Design review of the part built by this model. Coordinates are the model's own, in mm. A direction names the side the tool comes from. Coordinates: 2 decimals unless noted, no trailing zeros. Write each loop counter-clockwise with the first axis right and the second up, starting at its lowest first coordinate (ties: lowest second). Pieces come first, ordered by that corner, then holes. Notation, with made-up numbers: (63.25, 18) -> (84.25, 18) arc R21 ccw to (84.25, 43) -> close; hole circle Ø1 at (81, 89). An arc over 180 degrees is marked (long way). Return JSON: item names as keys, results as strings. Group by question number.
from build123d import *

# Parameters (mm, degrees)
CYLINDER095_R      = 1.5
CYLINDER095_DEPTH  = 21
CYLINDER094_R      = 1.5
CYLINDER094_DEPTH  = 21
CYLINDER085_R      = 1.5
CYLINDER085_DEPTH  = 12
CYLINDER088_R      = 3
CYLINDER088_DEPTH  = 1
CYLINDER089_R      = 3
CYLINDER089_DEPTH  = 1
CYLINDER087_R      = 5.5
CYLINDER087_DEPTH  = 4
CYLINDER086_R      = 5.5
CYLINDER086_DEPTH  = 4
BOX406008013_W     = 15
BOX406008013_H     = 29
BOX406008013_DEPTH = 18
CHAMFER_SIZE       = 0.5
CHAMFER001_SIZE    = 0.5


with BuildPart() as cylinder095:
    # Cylinder095 → Cylinder095 (new body)
    with BuildSketch(Plane(origin=(3, -13, -4), x_dir=(1, 0, 0), z_dir=(0, -1, 0))):
        Circle(CYLINDER095_R)
    extrude(amount=CYLINDER095_DEPTH)


with BuildPart() as fusion103077013004017014:
    # Cylinder094 → Cylinder094 (new body)
    with BuildSketch(Plane(origin=(-3, -13, -14), x_dir=(1, 0, 0), z_dir=(0, -1, 0))):
        Circle(CYLINDER094_R)
    extrude(amount=CYLINDER094_DEPTH)

    # Fusion103077013004017014: union Cylinder095
    add(cylinder095.part)


with BuildPart() as cylinder081:
    # Cylinder085 → Cylinder085 (new body)
    with BuildSketch(Plane.XY.offset(-14)):
        Circle(CYLINDER085_R)
    extrude(amount=CYLINDER085_DEPTH)


with BuildPart() as cylinder082:
    # Cylinder088 → Cylinder088 (new body)
    with BuildSketch(Plane.XY.offset(-5)):
        Circle(CYLINDER088_R)
    extrude(amount=CYLINDER088_DEPTH)


with BuildPart() as fusion103077013004017009:
    # Cylinder089 → Cylinder089 (new body)
    with BuildSketch(Plane.XY.offset(-14)):
        Circle(CYLINDER089_R)
    extrude(amount=CYLINDER089_DEPTH)

    # Fusion103077013004017009: union Cylinder082
    add(cylinder082.part)


with BuildPart() as f_623_bearing003:
    # Cylinder087 → Cylinder087 (new body)
    with BuildSketch(Plane.XY.offset(-18)):
        Circle(CYLINDER087_R)
    extrude(amount=CYLINDER087_DEPTH)


with BuildPart() as f_623_bearing_holes:
    # Cylinder086 → Cylinder086 (new body)
    with BuildSketch(Plane.XY.offset(-4)):
        Circle(CYLINDER086_R)
    extrude(amount=CYLINDER086_DEPTH)

    # Fusion103077013004017008: union 623 Bearing003
    add(f_623_bearing003.part)


with BuildPart() as bearing_mount_end:
    # Box406008013 → Box406008013 (new body)
    with BuildSketch(Plane(origin=(-7.5, -22, -18), x_dir=(1, 0, 0), z_dir=(0, 0, 1))):
        with Locations((7.5, 14.5)):
            Rectangle(BOX406008013_W, BOX406008013_H)
    extrude(amount=BOX406008013_DEPTH)

    # Cut070: cut 623 Bearing Holes
    add(f_623_bearing_holes.part, mode=Mode.SUBTRACT)

    # Cut071: cut Fusion103077013004017009
    add(fusion103077013004017009.part, mode=Mode.SUBTRACT)

    # Cut072: cut Cylinder081
    add(cylinder081.part, mode=Mode.SUBTRACT)

    # Chamfer
    chamfer_edges = [bearing_mount_end.edges().sort_by_distance(p)[0] for p in [
        (-3, 0, -5),
    ]]
    chamfer(chamfer_edges, length=CHAMFER_SIZE)

    # Chamfer001
    chamfer001_edges = [bearing_mount_end.edges().sort_by_distance(p)[0] for p in [
        (-3, 0, -13),
    ]]
    chamfer(chamfer001_edges, length=CHAMFER001_SIZE)

    # Cut078: cut Fusion103077013004017014
    add(fusion103077013004017014.part, mode=Mode.SUBTRACT)


solid = bearing_mount_end.part
Q1. We need section A-A on y = 0. Write out the cut boundary in (x, z), plus the area to 4 significant figures.
Q2. We need section C-C on z = -3. Write out the cut boundary in (x, y), plus the area to 3 significant figures.
Q3. We need section D-D on z = -7.25. Write out the cut boundary in (x, y), plus the area to 3 significant figures.
Q4. For faces 1 (the flat face through (0, -11, 0)), 2 (the flat face through (2.4, -2.4, -14)), 3 (the flat face through (-3, -13, -14)), 4 (the flat face through (2.4, -2.4, -4)), list the 3-axis set-ups (+Z, -Z, +X, -X, +Y, -Y) from which the entire face can be reached by the end or side of a thin tool; tool diameter is ignored.
Q5. Wall thickness on L1, parallel to Z at x = -3, y = -20.25; L2, parallel to X at y = -18.25, z = -14; L3, parallel to X at y = -15.25, z = -4: over which ranges is each line inside the solid? List them lowest first.
Q6. The part is to be moulded in two halves that separate along X. For faces 5 (the flat face through (-7.5, -8, -9)), 6 (the flat face through (0, -22, -9)), 7 (the cylindrical face through (-1.5, 0.07, -9.06)), 8 (the flat face through (7.5, -8, -9)), say which applies: +X half, -X half, draft (parallel to the pull), parting line (faces both ways), or undercut.
Q7. For P1, Ø5.5, axis at x = 0, y = -1, coming from the -Z side; P2, Ø5.5, axis at x = 1, y = 0, coming from the +Z side; P3, Ø0.9, axis at x = 3.5, z = -4.5, coming from the -Y side, all flat-tipped, find the tip position at first contact; note any pin that passes through.
Q8. We need section B-B on x = 0. Write out the cut boundary in (y, z).
Findings below:
{
 "1": {"outline": "(-7.5, -18) -> (-5.5, -18) -> (-5.5, -14) -> (-3, -14) -> (-3, -13.5) -> (-2.5, -13) -> (-1.5, -13) -> (-1.5, -5) -> (-2.5, -5) -> (-3, -4.5) -> (-3, -4) -> (-5.5, -4) -> (-5.5, 0) -> (-7.5, 0) -> close; (1.5, -13) -> (2.5, -13) -> (3, -13.5) -> (3, -14) -> (5.5, -14) -> (5.5, -18) -> (7.5, -18) -> (7.5, 0) -> (5.5, 0) -> (5.5, -4) -> (3, -4) -> (3, -4.5) -> (2.5, -5) -> (1.5, -5) -> close", "area": "146.5 mm^2"},
 "2": {"outline": "(-7.5, -22) -> (1.88, -22) -> (1.88, -13) -> (4.12, -13) -> (4.12, -22) -> (7.5, -22) -> (7.5, 7) -> (-7.5, 7) -> close; hole circle Ø11 at (0, 0)", "area": "320 mm^2"},
 "3": {"outline": "(-7.5, -22) -> (7.5, -22) -> (7.5, 7) -> (-7.5, 7) -> close; hole circle Ø3 at (0, 0)", "area": "428 mm^2"},
 "4": {"face 1": "+Z, +X, -X, +Y, -Y", "face 2": "-Z", "face 3": "-Y", "face 4": "+Z"},
 "5": {"L1": "z = -18 to -15.5, -12.5 to 0", "L2": "x = -7.5 to -4.5, -1.5 to 7.5", "L3": "x = -7.5 to 1.5, 4.5 to 7.5"},
 "6": {"face 5": "-X half", "face 6": "draft", "face 7": "undercut", "face 8": "+X half"},
 "7": {"P1": "stops at z = -14", "P2": "stops at z = -4", "P3": "stops at y = -13"},
 "8": {"outline": "(-22, -18) -> (-5.5, -18) -> (-5.5, -14) -> (-3, -14) -> (-3, -13.5) -> (-2.5, -13) -> (-1.5, -13) -> (-1.5, -5) -> (-2.5, -5) -> (-3, -4.5) -> (-3, -4) -> (-5.5, -4) -> (-5.5, 0) -> (-22, 0) -> close; (1.5, -13) -> (2.5, -13) -> (3, -13.5) -> (3, -14) -> (5.5, -14) -> (5.5, -18) -> (7, -18) -> (7, 0) -> (5.5, 0) -> (5.5, -4) -> (3, -4) -> (3, -4.5) -> (2.5, -5) -> (1.5, -5) -> close"}
}
